The listing builds one solid part. Answer for the finished solid, in the listing's coordinates (mm). A direction names the side the tool comes from. Coordinates: 2 decimals unless noted, no trailing zeros. Write each loop counter-clockwise with the first axis right and the second up, starting at its lowest first coordinate (ties: lowest second). Pieces come first, ordered by that corner, then holes.
(1) Straight lines are drawn through the part: line 1 (Z direction, x = 16.5, y = 7.5); line 2 (Y direction, x = 7, z = -0.3); line 3 (Y direction, x = 0, z = 0.25). For each, find the intervals that lie inside material, in ascending order.
(2) Given P1, Ø2, axis at y = 16, z = 1, coming from the -X side (3 decimals); P2, Ø4, axis at x = -11, y = 14.5, coming from the +Z side, each flat-ended and moving along its own axis, determine where each tip first touches the part or whether it passes through.
(3) Which of the six approach directions +Z, -Z, +X, -X, +Y, -Y give full straight-line access (tool end or side, diameter ignored) to faces 1 (the flat face through (-10, 14, -1.1)), 2 (the flat face through (3, -10, -2.65))?
(4) For a pull along Y with two mould halves and no side action, classify faces 3 (the cylindrical face through (4.38, -8.43, -0.03)), 4 (the flat face through (10, 14, 1.1)) as +Y half, -Y half, draft (parallel to the pull), parting line (faces both ways), or undercut.
(5) The part is cut by section A-A on y = 0. Determine the outline of the cut face in (x, z), plus the area to 3 significant figures.
from build123d import *

# Parameters (mm, degrees)
F0_R     = 25
F0_R_2   = 9.5
F1_DEPTH = 2.65
F4_R     = 1.5
F5_SIZE  = 0.5


with BuildPart() as f1:
    # F0 (on Top) → F1 (new body, symmetric)
    with BuildSketch(Plane.XY):
        Circle(F0_R)
        Circle(F0_R_2, mode=Mode.SUBTRACT)
    extrude(amount=F1_DEPTH, both=True)

    # F2 (on Front) → F3 (revolve, cut)
    with BuildSketch(Plane.XZ):
        Polygon((42.872044, 12.488453), (15.5, 2.65), (15.5, 1.1), (23.094744, 1.1), (25, 0), (23.094744, -1.1), (15.5, -1.1), (15.5, -2.672665), (42.872044, -11.621938), align=None)
    revolve(axis=Axis((0, 0, -3.257056), (0, 0, -1)), mode=Mode.SUBTRACT)

    # F4
    f4_edges = [f1.edges().sort_by_distance(p)[0] for p in [
        (-15.5, 0, 1.1),
        (-15.5, 0, -1.1),
    ]]
    fillet(f4_edges, radius=F4_R)

    # F5
    f5_edges = [f1.edges().sort_by_distance(p)[0] for p in [
        (-9.5, 0, 2.65),
        (-9.5, 0, -2.65),
    ]]
    chamfer(f5_edges, length=F5_SIZE)


solid = f1.part
Model answer:
1. line 1: z = -1.1 to 1.1
1. line 2: y = -23.46 to -6.42, 6.42 to 23.46
1. line 3: y = -24.57 to -9.5, 9.5 to 24.57
2. P1: stops at x = -19.355
2. P2: stops at z = 1.33
3. face 1: -Z
3. face 2: -Z, +X, -X, +Y, -Y
4. face 3: undercut
4. face 4: draft
5. outline: (-25, 0) - (-23.09, -1.1) - (-17, -1.1) arc R1.5 cw to (-15.5, -2.6) - (-15.5, -2.65) - (-10, -2.65) - (-9.5, -2.15) - (-9.5, 2.15) - (-10, 2.65) - (-15.5, 2.65) - (-15.5, 2.6) arc R1.5 cw to (-17, 1.1) - (-23.09, 1.1) - close; (9.5, -2.15) - (10, -2.65) - (15.5, -2.65) - (15.5, -2.6) arc R1.5 cw to (17, -1.1) - (23.09, -1.1) - (25, 0) - (23.09, 1.1) - (17, 1.1) arc R1.5 cw to (15.5, 2.6) - (15.5, 2.65) - (10, 2.65) - (9.5, 2.15) - close
5. area: 103 mm2
